```python
from build123d import *

# Parameters (mm, degrees)
F0_R     = 1.5
F0_R_2   = 3
F1_DEPTH = 3
F2_R     = 10


# Not quite as in the source:
# - a feature names something its author has since deleted; it is built from what else it names


with BuildPart() as f1:
    # F0 (on Front) → F1 (new body)
    with BuildSketch(Plane.XZ):
        Polygon((-197, 0), (0, 0), (0, 25), (-31.75, 25), (-63.5, 25), (-76.0906166883, 25), (-120.9093833117, 25), (-133.5, 25), (-165.25, 25), (-197, 25), align=None)
        with Locations((-184, 12.5)):
            Circle(F0_R, mode=Mode.SUBTRACT)
        with Locations((-165.25, 12.5)):
            Circle(F0_R, mode=Mode.SUBTRACT)
        with Locations((-146.5, 12.5)):
            Circle(F0_R, mode=Mode.SUBTRACT)
        with Locations((-98.5, 12.5)):
            Circle(F0_R_2, mode=Mode.SUBTRACT)
        with Locations((-50.5, 12.5)):
            Circle(F0_R, mode=Mode.SUBTRACT)
        with Locations((-31.75, 12.5)):
            Circle(F0_R, mode=Mode.SUBTRACT)
        with Locations((-13, 12.5)):
            Circle(F0_R, mode=Mode.SUBTRACT)
        with BuildLine():
            Line((-63.5, 25), (-31.75, 25))
            ThreePointArc((-31.75, 25), (-40.2438467547, 27.571729868), (-45.8846153846, 34.4230769231))
            ThreePointArc((-45.8846153846, 34.4230769231), (-49.720477364, 37.4388606439), (-54.2987189286, 35.7511128097))
            Line((-54.2987189286, 35.7511128097), (-63.5, 25))
        make_face()
        with Locations((-50.5, 32.5)):
            Circle(F0_R, mode=Mode.SUBTRACT)
        with BuildLine():
            Line((-31.75, 25), (0, 25))
            Line((0, 25), (-9.2012810714, 35.7511128097))
            ThreePointArc((-9.2012810714, 35.7511128097), (-13.779522636, 37.4388606439), (-17.6153846154, 34.4230769231))
            ThreePointArc((-17.6153846154, 34.4230769231), (-23.2561532453, 27.571729868), (-31.75, 25))
        make_face()
        with Locations((-13, 32.5)):
            Circle(F0_R, mode=Mode.SUBTRACT)
        with BuildLine():
            Line((-187.7987189286, 35.7511128097), (-197, 25))
            Line((-197, 25), (-165.25, 25))
            ThreePointArc((-165.25, 25), (-173.7438467547, 27.571729868), (-179.3846153846, 34.4230769231))
            ThreePointArc((-179.3846153846, 34.4230769231), (-183.220477364, 37.4388606439), (-187.7987189286, 35.7511128097))
        make_face()
        with Locations((-184, 32.5)):
            Circle(F0_R, mode=Mode.SUBTRACT)
        with BuildLine():
            ThreePointArc((-151.1153846154, 34.4230769231), (-156.7561532453, 27.571729868), (-165.25, 25))
            Line((-165.25, 25), (-133.5, 25))
            Line((-133.5, 25), (-142.7012810714, 35.7511128097))
            ThreePointArc((-142.7012810714, 35.7511128097), (-147.279522636, 37.4388606439), (-151.1153846154, 34.4230769231))
        make_face()
        with Locations((-146.5, 32.5)):
            Circle(F0_R, mode=Mode.SUBTRACT)
        with BuildLine():
            Line((-120.9093833117, 25), (-76.0906166883, 25))
            Line((-76.0906166883, 25), (-85.9197777844, 36.7139380484))
            ThreePointArc((-85.9197777844, 36.7139380484), (-87.6369086913, 38.0315389352), (-89.75, 38.5))
            Line((-89.75, 38.5), (-107.25, 38.5))
            ThreePointArc((-107.25, 38.5), (-109.3630913087, 38.0315389352), (-111.0802222156, 36.7139380484))
            Line((-111.0802222156, 36.7139380484), (-120.9093833117, 25))
        make_face()
        with Locations((-107.25, 33.5)):
            Circle(F0_R, mode=Mode.SUBTRACT)
        with Locations((-89.75, 33.5)):
            Circle(F0_R, mode=Mode.SUBTRACT)
    extrude(amount=F1_DEPTH)

    # F2
    f2_edges = [f1.edges().sort_by_distance(p)[0] for p in [
        (0, -1.5, 25),
        (-197, -1.5, 25),
        (-133.5, -1.5, 25),
        (-63.5, -1.5, 25),
        (-120.909383, -1.5, 25),
        (-76.090617, -1.5, 25),
    ]]
    fillet(f2_edges, radius=F2_R)


solid = f1.part
```
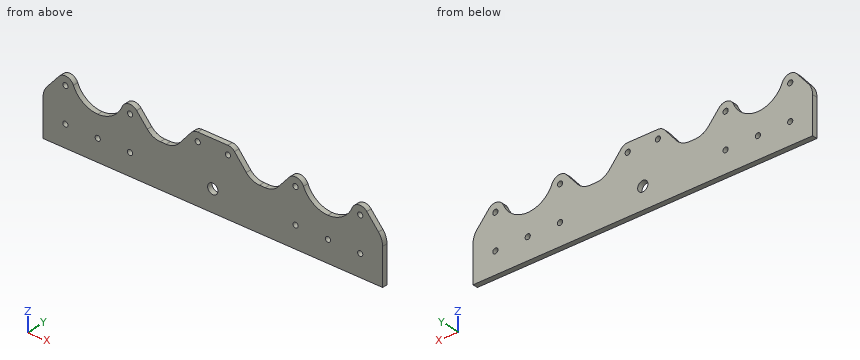
Could you check a few things on this model? Use its own coordinates, in mm. Round coordinates to 2 decimals unless told otherwise and drop trailing zeros. Loops run counter-clockwise (first coordinate to the right, second up) from the corner with the lowest first, then second, coordinate; pieces in that order, holes last. Notation, with made-up numbers: M 28.5,54 L 79.5,54 A20 ccw 79.5,58 Z; hole C -37.75,22 d2. An arc over 180 degrees is marked long. Put each result on its own line as item: value.
Q1. Imagine slicing it at A-A (y = -1.55). State how many separate pieces and enclosed holes the cut face has, then the cut area to 3 significant figures.
Check result:
separate pieces: 1
enclosed holes: 13
area: 6,010 mm2
Q2. For pin 1 (0.9 mm diameter, centred on x = -128, y = -1.5, fed in from +Z); pin 2 (8 mm diameter, centred on x = -70, z = 28, fed in from -Y), each with a flat end and sliding along its axis, tell me the tip position at first contact or that it passes through.
Check result:
pin 1: z = 25
pin 2: y = -3
Q3. I need wall thicknesses on probe 1 along Z at (x, y) = (-184, -1.5); probe 2 along Z at (x, y) = (-165.25, -1.1); probe 3 along Z at (x, y) = (-107.25, -0.8). Which ranges of each line are inside material? Lowest first, please.
Check result:
probe 1: 0 to 11, 14 to 31, 34 to 37.5
probe 2: 0 to 11, 14 to 25
probe 3: 0 to 32, 35 to 38.5
Q4. Imagine slicing it at B-B (x = -139). Write out the boundary of the cut face in (y, z), then the cut area to 3 significant figures.
Check result:
outline: M -3,0 L 0,0 L 0,31.43 L -3,31.43 Z
area: 94.3 mm2
Q5. Imagine slicing it at C-C (x = -63.5). Write out the boundary of the cut face in (y, z), then the cut area to 3 significant figures.
Check result:
outline: M -3,0 L 0,0 L 0,26.12 L -3,26.12 Z
area: 78.4 mm2
